```python
from build123d import *

# Parameters (mm, degrees)
SKETCH1_W            = 62
SKETCH1_H            = 9
BOSS_EXTRUDE1_DEPTH  = 1
BOSS_EXTRUDE2_DEPTH  = 3
SKETCH3_W            = 5
SKETCH3_H            = 1.8
CUT_EXTRUDE1_DEPTH   = 3
SKETCH4_R            = 1
CUT_EXTRUDE2_DEPTH   = 63.721607122
SKETCH5_W            = 4
SKETCH5_H            = 5
BOSS_EXTRUDE4_DEPTH  = 1
BOSS_EXTRUDE5_DEPTH  = 1
SKETCH7_R            = 2.125973312
BOSS_EXTRUDE6_DEPTH  = 0.3
BOSS_EXTRUDE7_DEPTH  = 1
SKETCH9_R            = 4
BOSS_EXTRUDE8_DEPTH  = 2
SKETCH10_R           = 2.014523047
BOSS_EXTRUDE9_DEPTH  = 3
SKETCH11_R           = 5
BOSS_EXTRUDE10_DEPTH = 3
CUT_EXTRUDE3_START   = -1
SKETCH12_R           = 4
CUT_EXTRUDE3_DEPTH   = 1
SKETCH13_R           = 0.341110464
CUT_EXTRUDE4_DEPTH   = 0.3


with BuildPart() as part:
    # Sketch1 → Boss-Extrude1 (new body)
    with BuildSketch(Plane(origin=(0, 0, 0), x_dir=(1, 0, 0), z_dir=(0, 1, 0))):
        with Locations((31, 4.5)):
            Rectangle(SKETCH1_W, SKETCH1_H)
    extrude(amount=BOSS_EXTRUDE1_DEPTH)

    # Sketch2 → Boss-Extrude2 (add)
    with BuildSketch(Plane(origin=(0, 1, 0), x_dir=(1, 0, 0), z_dir=(0, 1, 0))):
        Polygon((62, 4.5), (62, 8), (58, 8), (58, 1), (62, 1), align=None)
    extrude(amount=BOSS_EXTRUDE2_DEPTH)

    # Sketch3 → Cut-Extrude1 (cut)
    with BuildSketch(Plane(origin=(62, 0, 0), x_dir=(0, 0, -1), z_dir=(1, 0, 0))):
        with Locations((4.5, 2.5)):
            Rectangle(SKETCH3_W, SKETCH3_H)
    extrude(amount=-CUT_EXTRUDE1_DEPTH, mode=Mode.SUBTRACT)

    # Sketch4 → Cut-Extrude2 (cut, through all)
    with BuildSketch(Plane(origin=(0, 1, 0), x_dir=(1, 0, 0), z_dir=(0, 1, 0))):
        with Locations(Location((2.2, 7.3, 0), (0, 0, 270))):
            Circle(SKETCH4_R)
        with Locations(Location((2.2, 1.7, 0), (0, 0, 270))):
            Circle(SKETCH4_R)
        with Locations(Location((52, 7, 0), (0, 0, 270))):
            Circle(SKETCH4_R)
    extrude(amount=-CUT_EXTRUDE2_DEPTH, mode=Mode.SUBTRACT)

    # Sketch5 → Boss-Extrude4 (add)
    with BuildSketch(Plane(origin=(0, 1, 0), x_dir=(1, 0, 0), z_dir=(0, 1, 0))):
        with Locations((46, 5.5)):
            Rectangle(SKETCH5_W, SKETCH5_H)
    extrude(amount=BOSS_EXTRUDE4_DEPTH)

    # Sketch6 → Boss-Extrude5 (add)
    with BuildSketch(Plane(origin=(0, 1, 0), x_dir=(1, 0, 0), z_dir=(0, 1, 0))):
        Polygon((10, 2), (10, 4.5), (10, 7), (15, 7), (15, 4.5), (15, 2), align=None)
    extrude(amount=BOSS_EXTRUDE5_DEPTH)

    # Sketch7 → Boss-Extrude6 (add)
    with BuildSketch(Plane(origin=(0, 2, 0), x_dir=(1, 0, 0), z_dir=(0, 1, 0))):
        with Locations(Location((12.5, 4.5, 0), (0, 0, 270))):
            Circle(SKETCH7_R)
    extrude(amount=BOSS_EXTRUDE6_DEPTH)

    # Sketch8 → Boss-Extrude7 (add)
    with BuildSketch(Plane(origin=(0, 1, 0), x_dir=(1, 0, 0), z_dir=(0, 1, 0))):
        Polygon((36, 8.5), (28, 8.5), (28, 4.5), (28, 0.5), (36, 0.5), (36, 4.5), align=None)
    extrude(amount=BOSS_EXTRUDE7_DEPTH)

    # Sketch9 → Boss-Extrude8 (add)
    with BuildSketch(Plane(origin=(0, 2, 0), x_dir=(1, 0, 0), z_dir=(0, 1, 0))):
        with Locations(Location((32, 4.5, 0), (0, 0, 270))):
            Circle(SKETCH9_R)
    extrude(amount=BOSS_EXTRUDE8_DEPTH)

    # Sketch10 → Boss-Extrude9 (add)
    with BuildSketch(Plane(origin=(0, 4, 0), x_dir=(1, 0, 0), z_dir=(0, 1, 0))):
        with Locations(Location((32, 4.5, 0), (0, 0, 270))):
            Circle(SKETCH10_R)
    extrude(amount=BOSS_EXTRUDE9_DEPTH)

    # Sketch11 → Boss-Extrude10 (add)
    with BuildSketch(Plane(origin=(0, 7, 0), x_dir=(1, 0, 0), z_dir=(0, 1, 0))):
        with Locations(Location((32, 4.5, 0), (0, 0, 270))):
            Circle(SKETCH11_R)
    extrude(amount=BOSS_EXTRUDE10_DEPTH)

    # Sketch12 → Cut-Extrude3 (cut)
    with BuildSketch(Plane(origin=(0, 10, 0), x_dir=(1, 0, 0), z_dir=(0, 1, 0)).offset(CUT_EXTRUDE3_START)):
        with Locations(Location((32, 4.5, 0), (0, 0, 270))):
            Circle(SKETCH12_R)
    extrude(amount=CUT_EXTRUDE3_DEPTH, mode=Mode.SUBTRACT)

    # Sketch13 → Cut-Extrude4 (cut)
    with BuildSketch(Plane(origin=(0, 2, 0), x_dir=(1, 0, 0), z_dir=(0, 1, 0))):
        with Locations(Location((46, 3.845478616, 0), (0, 0, 270))):
            Circle(SKETCH13_R)
    extrude(amount=-CUT_EXTRUDE4_DEPTH, mode=Mode.SUBTRACT)


solid = part.part
```
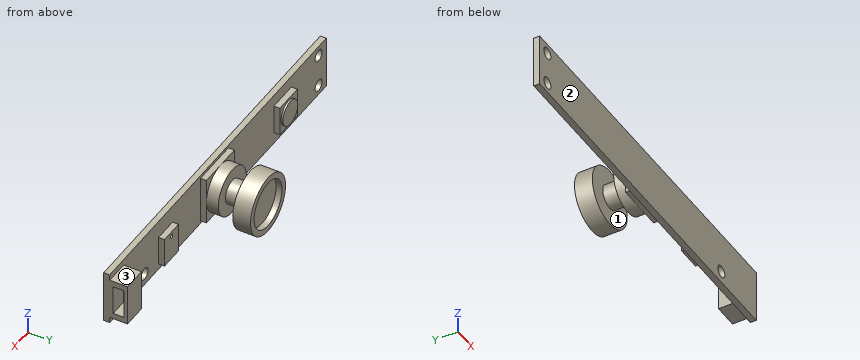
The model under review builds one solid part; all positions refer to its coordinate system, in mm. Face numbers are marked on the shaded views. Give positions to 0.01 mm unless a question says otherwise; leave off trailing zeros. Write each loop counter-clockwise with the first axis right and the second up, starting at its lowest first coordinate (ties: lowest second). Pieces come first, ordered by that corner, then holes. Notation, with made-up numbers: M 76,39 L 96,39 A23 cw 96,72 Z; hole C -19.5,30 d9. An arc over 180 degrees is marked long. Write item = value, one per line. Start each with the question number.
Q1. We need section A-A (x = 52). State the section outline as (y, z) points, plus the area to 3 significant figures.
Q2. For line 1 (X direction, y = 1.5, z = -5.25); line 2 (X direction, y = 1.75, z = -4.25); line 3 (Z direction, x = 46, y = 1.95), list the stretches that pass through material, from the lowest coordinate up.
Q3. We need section C-C (x = 12.5). State the section outline as (y, z) points.
Q4. Clearance check with flat-ended pins moving along their axes: pin 1 (1.4 mm diameter, centred on x = 61, y = 2.5, fed in from -Z); pin 2 (2.5 mm diameter, centred on x = 60.5, y = 2, fed in from +Z); pin 3 (3 mm diameter, centred on x = 41.5, z = -2, fed in from +Y); pin 4 (1.6 mm diameter, centred on x = 2.2, z = -1.7, fed in from +Y). State where each tip first meets the part, or that it passes through.
Q5. Mouldability with a two-part tool opening along Y and no side actions: class the marked faces 1, 2 and 3 as released by +Y, released by -Y, zero draft, split by the parting line, or undercut.
Q6. We need section D-D (y = 5.25). State the section outline as (x, z) points.
Q7. We need section B-B (x = 2.2). State the section outline as (y, z) points, plus the area to 3 significant figures.
Result set:
q1.outline = M 0,-9 L 1,-9 L 1,-8 L 0,-8 Z; M 0,-6 L 1,-6 L 1,0 L 0,0 Z
q1.area = 7.00 mm2
q2.line_1 = 10 to 15, 28 to 36, 44 to 48, 58 to 62
q2.line_2 = 10 to 15, 28 to 36, 44 to 48, 58 to 59
q2.line_3 = -8 to -4.19, -3.5 to -3
q3.outline = M 0,-9 L 1,-9 L 1,-7 L 2,-7 L 2,-6.63 L 2.3,-6.63 L 2.3,-2.37 L 2,-2.37 L 2,-2 L 1,-2 L 1,0 L 0,0 Z
q4.pin_1 = -8
q4.pin_2 = 0
q4.pin_3 = 1
q4.pin_4 = through
q5.face_1 = undercut
q5.face_2 = released by -Y
q5.face_3 = zero draft
q6.outline = C 32,-4.5 d4.03
q7.outline = M 0,-9 L 1,-9 L 1,-8.3 L 0,-8.3 Z; M 0,-6.3 L 1,-6.3 L 1,-2.7 L 0,-2.7 Z; M 0,-0.7 L 1,-0.7 L 1,0 L 0,0 Z
q7.area = 5.00 mm2
